The figure shows three views and two pictorial views of one solid part (mm, origin at its lowest corner). Answer the questions. A direction names the side the tool comes from. Coordinates: 2 decimals unless noted, no trailing zeros. Loops run counter-clockwise (first coordinate to the right, second up) from the corner with the lowest first, then second, coordinate; pieces in that order, holes last. Notation, with made-up numbers: (-37.75, 63.5) -> (21.25, 63.5) arc R10 cw to (21.25, 75.5) -> close; hole circle Ø7 at (-38, 5.25). An arc over 180 degrees is marked (long way). Answer as a JSON object with one key per item and string values. Group by question number.
1) Consider probe 1 along Y at (x, z) = (20, 2.75) (3 decimals); probe 2 along Y at (x, z) = (21, 10.25) (3 decimals); probe 3 along Z at (x, y) = (16.5, 32). Determine where each line is inside the solid, lowest interval first. Write a range as [from, to].
2) Flat-ended cylindrical pins translate along their axes: P1, Ø1, axis at y = 24, z = 0.5, coming from the -X side; P2, Ø2, axis at x = 17.5, y = 4.5, coming from the +Z side (3 decimals); P3, Ø1.5, axis at y = 7.5, z = 5, coming from the -X side; P4, Ø1.5, axis at x = 20, z = 10, coming from the +Y side (3 decimals). Find the tip coordinate at first contact, or state that the pin passes through.
3) Section B-B, the plane x = 12 is taken. Give the vertices of the cut face in (y, z) (3 decimals).
4) Section A-A, the plane y = 16.5 is taken. Give the vertices of the cut face in (x, z) (3 decimals), plus the area to 3 significant figures.
5) Section C-C, the plane z = 1.75 is taken. Give the vertices of the cut face in (x, y) (3 decimals).
6) Determine the mould class of the marked faces 1, 2 and 3 for opening direction Y: released by +Y, released by -Y, zero draft, split by the parting line, or undercut.
7) Section D-D, the plane y = 8 is taken. Give the vertices of the cut face in (x, z) (3 decimals), plus the area to 3 significant figures.
8) Which of the six approach directions +Z, -Z, +X, -X, +Y, -Y give full straight-line access (tool end or side, diameter ignored) to the marked faces 4 and 5?
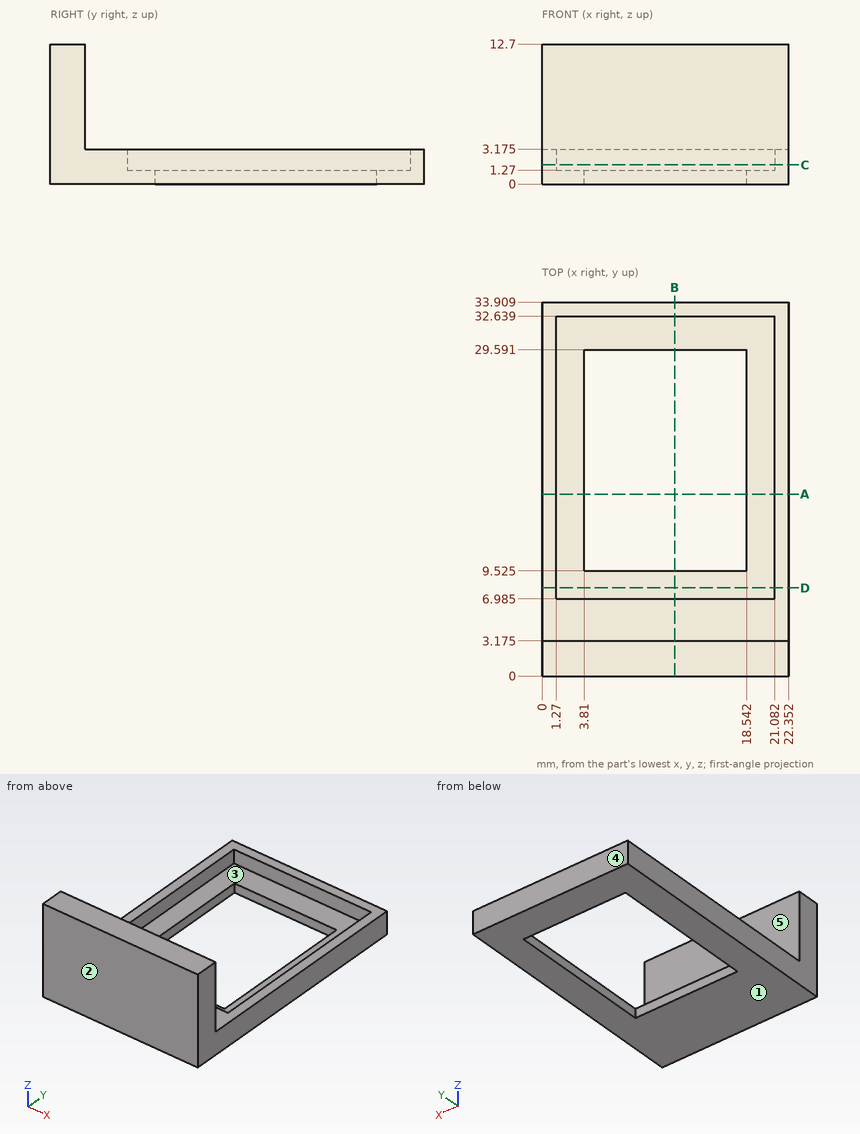
Determined:
{
 "1": {"probe 1": "[0, 6.985], [32.639, 33.909]", "probe 2": "[0, 3.175]", "probe 3": "[0, 1.27]"},
 "2": {"P1": "x = 0", "P2": "z = 3.175", "P3": "through", "P4": "y = 3.175"},
 "3": {"outline": "(0, 0) -> (9.525, 0) -> (9.525, 1.27) -> (6.985, 1.27) -> (6.985, 3.175) -> (3.175, 3.175) -> (3.175, 12.7) -> (0, 12.7) -> close; (29.591, 0) -> (33.909, 0) -> (33.909, 3.175) -> (32.639, 3.175) -> (32.639, 1.27) -> (29.591, 1.27) -> close"},
 "4": {"outline": "(0, 0) -> (3.81, 0) -> (3.81, 1.27) -> (1.27, 1.27) -> (1.27, 3.175) -> (0, 3.175) -> close; (18.542, 0) -> (22.352, 0) -> (22.352, 3.175) -> (21.082, 3.175) -> (21.082, 1.27) -> (18.542, 1.27) -> close", "area": "14.5 mm²"},
 "5": {"outline": "(0, 0) -> (22.352, 0) -> (22.352, 33.909) -> (0, 33.909) -> close; hole (1.27, 6.985) -> (21.082, 6.985) -> (21.082, 32.639) -> (1.27, 32.639) -> close"},
 "6": {"face 1": "zero draft", "face 2": "released by -Y", "face 3": "undercut"},
 "7": {"outline": "(0, 0) -> (22.352, 0) -> (22.352, 3.175) -> (21.082, 3.175) -> (21.082, 1.27) -> (1.27, 1.27) -> (1.27, 3.175) -> (0, 3.175) -> close", "area": "33.2 mm²"},
 "8": {"face 4": "+Z, -Z, +X, -X, +Y", "face 5": "+Z, +X, -X, +Y"}
}
